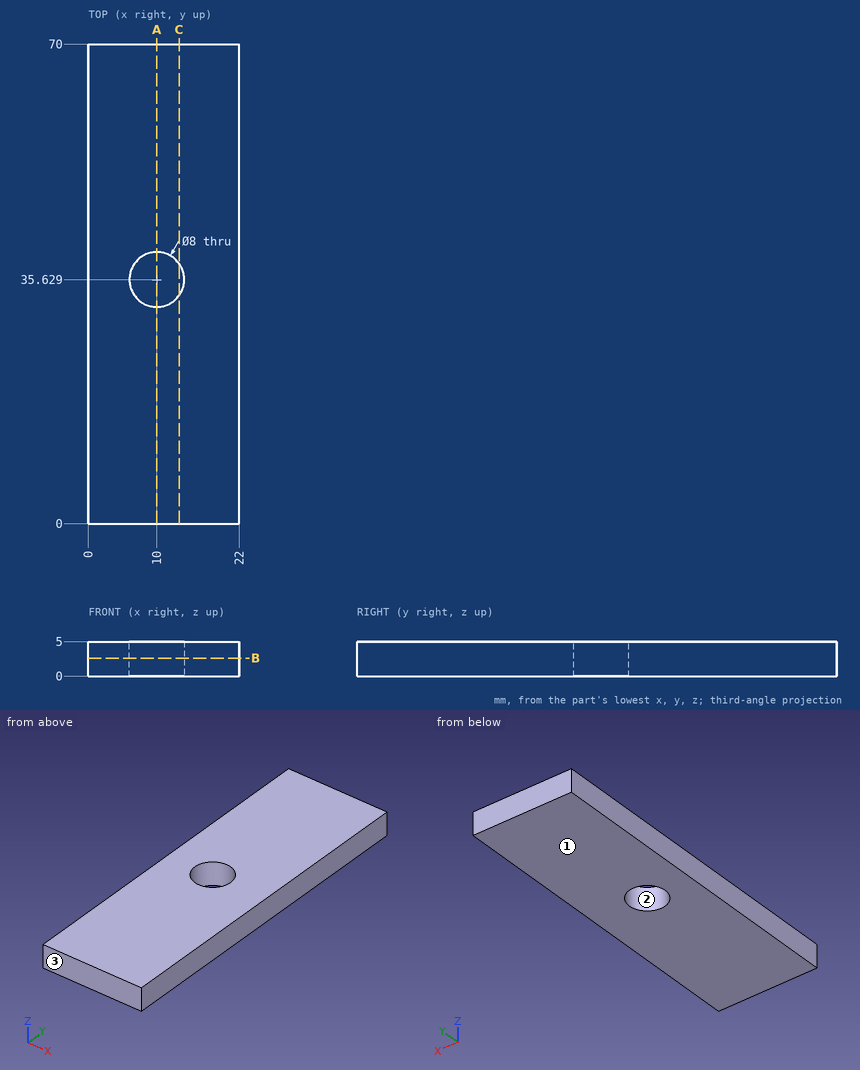
Verification items for this drawing (mm, ordinates from the low corner). Coordinates: 2 decimals unless noted, no trailing zeros. Loops run counter-clockwise (first coordinate to the right, second up) from the corner with the lowest first, then second, coordinate; pieces in that order, holes last. Notation, with made-up numbers: (4, 75) -> (10, 75) arc R33 ccw to (10, 110) -> close; hole circle Ø8 at (14, -21). An arc over 180 degrees is marked (long way). Answer in a Markdown table with one row per item. Add a question column.
1. Material ranges on probe 1 along Y at (x, z) = (10.25, 0.5); probe 2 along X at (y, z) = (32, 0.85) (1 decimal); probe 3 along Y at (x, z) = (7, 0.95) (1 decimal), recorded low to high. Write a range as [from, to].
2. Section check A-A, the plane x = 10. Enter the section's corners in (y, z), then the cut area to 3 significant figures.
3. Depth check by flat-ended pin: P1, Ø2, axis at x = 5.5, y = 10.5, coming from the -Z side. Enter the tip coordinate at first touch or a pass-through.
4. Section check B-B, the plane z = 2.6. Enter the section's corners in (x, y).
5. Draft check along Y on the marked faces 1, 2 and 3. Enter one of: +Y half, -Y half, draft (parallel to the pull), parting line (faces both ways), or undercut.
6. Section check C-C, the plane x = 13.25. Enter the section's corners in (y, z), then the cut area to 3 significant figures.
Derived:
| question | item | result |
|---|---|---|
| 1 | probe 1 | y = [0, 31.64], [39.62, 70] |
| 1 | probe 2 | x = [0, 8.3], [11.7, 22] |
| 1 | probe 3 | y = [0, 33], [38.3, 70] |
| 2 | outline | (0, 0) -> (31.63, 0) -> (31.63, 5) -> (0, 5) -> close; (39.63, 0) -> (70, 0) -> (70, 5) -> (39.63, 5) -> close |
| 2 | area | 310 mm² |
| 3 | P1 | stops at z = 0 |
| 4 | outline | (0, 0) -> (22, 0) -> (22, 70) -> (0, 70) -> close; hole circle Ø8 at (10, 35.63) |
| 5 | face 1 | draft |
| 5 | face 2 | undercut |
| 5 | face 3 | -Y half |
| 6 | outline | (0, 0) -> (33.3, 0) -> (33.3, 5) -> (0, 5) -> close; (37.96, 0) -> (70, 0) -> (70, 5) -> (37.96, 5) -> close |
| 6 | area | 327 mm² |
